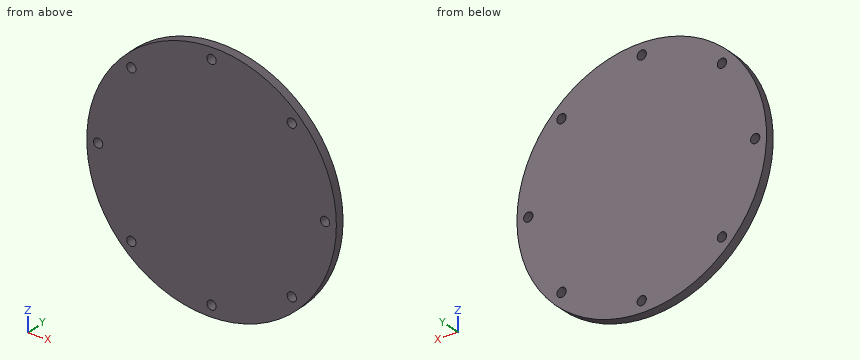
```python
from build123d import *

# Parameters (mm, degrees)
SKETCH1_R           = 26.95
SKETCH1_R_2         = 1
BOSS_EXTRUDE1_DEPTH = 2


with BuildPart() as part:
    # Sketch1 → Boss-Extrude1 (new body)
    with BuildSketch(Plane(origin=(0, 0, 0), x_dir=(1, 0, 0), z_dir=(0, 1, 0))):
        Circle(SKETCH1_R)
        with Locations((0, 24.5)):
            Circle(SKETCH1_R_2, mode=Mode.SUBTRACT)
        with Locations((17.324116139, 17.324116139)):
            Circle(SKETCH1_R_2, mode=Mode.SUBTRACT)
        with Locations((24.5, 0)):
            Circle(SKETCH1_R_2, mode=Mode.SUBTRACT)
        with Locations((17.324116139, -17.324116139)):
            Circle(SKETCH1_R_2, mode=Mode.SUBTRACT)
        with Locations((0, -24.5)):
            Circle(SKETCH1_R_2, mode=Mode.SUBTRACT)
        with Locations((-17.324116139, -17.324116139)):
            Circle(SKETCH1_R_2, mode=Mode.SUBTRACT)
        with Locations((-24.5, 0)):
            Circle(SKETCH1_R_2, mode=Mode.SUBTRACT)
        with Locations((-17.324116139, 17.324116139)):
            Circle(SKETCH1_R_2, mode=Mode.SUBTRACT)
    extrude(amount=BOSS_EXTRUDE1_DEPTH)


solid = part.part
```
Could you check a few things on this model? Use its own coordinates, in mm. Round coordinates to 2 decimals unless told otherwise and drop trailing zeros. Order: outer loops, then holes, each group sorted by start corner. A loop starts at its lowest first (then second) coordinate and runs counter-clockwise, first axis right, second up. Notation, with made-up numbers: (2.5, 69) -> (38.5, 69) arc R23 ccw to (38.5, 94) -> close; hole circle Ø10 at (66.25, 29.25). An arc over 180 degrees is marked (long way). One line per question, with ' | ' between items.
Q1. If we section it at C-C on z = -24.5: Write out the boundary of the cut face in (x, y), plus the area to 3 significant figures.
Computed values:
outline: (-11.23, 0) -> (-1, 0) -> (-1, 2) -> (-11.23, 2) -> close; (1, 0) -> (11.23, 0) -> (11.23, 2) -> (1, 2) -> close | area: 40.9 mm²
Q2. If we section it at A-A on z = 0: Write out the boundary of the cut face in (x, y).
Computed values:
outline: (-26.95, 0) -> (-25.5, 0) -> (-25.5, 2) -> (-26.95, 2) -> close; (-23.5, 0) -> (23.5, 0) -> (23.5, 2) -> (-23.5, 2) -> close; (25.5, 0) -> (26.95, 0) -> (26.95, 2) -> (25.5, 2) -> close
Q3. If I drill on line 1 (X direction, y = 1.3, z = 0); line 2 (X direction, y = 0.35, z = 17.5), over which ranges is the centre line in solid material (lowest first)? Write a range as from..to.
Computed values:
line 1: -26.95..-25.5, -23.5..23.5, 25.5..26.95 | line 2: -20.5..-18.31, -16.34..16.34, 18.31..20.5
Q4. If we section it at D-D on y = 0.8: Give the number of separate pieces and of enclosed holes in the cut face, plus the area to 3 significant figures.
Computed values:
separate pieces: 1 | enclosed holes: 8 | area: 2,260 mm²
Q5. If we section it at B-B on x = 0: Write out the boundary of the cut face in (y, z), plus the area to 3 significant figures.
Computed values:
outline: (0, -26.95) -> (2, -26.95) -> (2, -25.5) -> (0, -25.5) -> close; (0, -23.5) -> (2, -23.5) -> (2, 23.5) -> (0, 23.5) -> close; (0, 25.5) -> (2, 25.5) -> (2, 26.95) -> (0, 26.95) -> close | area: 99.8 mm²
